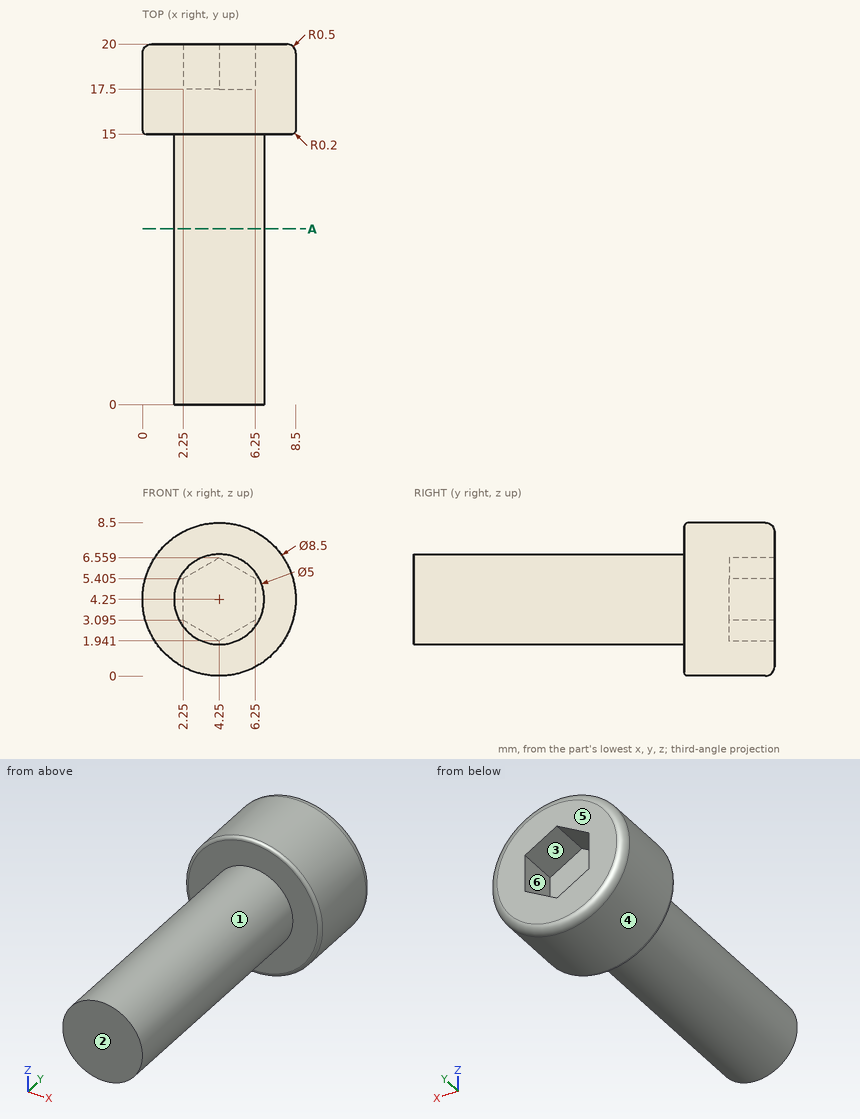
Could you check a few things on this drawing? It's one solid part, dimensions in mm from its lowest x, y, z. A direction names the side the tool comes from. Give positions to 0.01 mm unless a question says otherwise; leave off trailing zeros. Write each loop counter-clockwise with the first axis right and the second up, starting at its lowest first coordinate (ties: lowest second). Pieces come first, ordered by that corner, then holes. Notation, with made-up numbers: (31.25, 84) - (71.25, 84) arc R26 cw to (71.25, 113) - close; hole circle Ø5 at (20.25, -8.5). An arc over 180 degrees is marked (long way). Use CSV: the item, a comma, the result in double quotes. Start each with the question number.
Item 1: For the marked faces 1, 2 and 3, which set-ups out of +Z, -Z, +X, -X, +Y, -Y let a thin tool reach every point of the face, with its end or its side?
Item 2: I want a section at A-A, the plane y = 9.75. Please give me the cut outline in (x, z).
Item 3: If I drill on line 1 along Y through (x, z) = (3.5, 2.5); line 2 along Z through (x, y) = (2.75, 6); line 3 along Y through (x, z) = (6, 6.75), over which ranges is the centre line in solid material (lowest first)?
Item 4: If we mould it in two halves opening along Z, with no side actions, what happens to the marked faces 4, 5 and 6? For each: pulls with the +Z half, pulls with the -Z half, needs draft (parallel to the pull), parting line crosses it, or undercut.
Item 5: I'm going to push flat-ended pins straight in: pin 1 (4 mm diameter, centred on y = 8, z = 7.5, fed in from -X) (1 decimal); pin 2 (5 mm diameter, centred on y = 3, z = 3.5, fed in from -X); pin 3 (3 mm diameter, centred on x = 7, y = 3.5, fed in from -Z) (1 decimal). Where does each tip first touch, or does it pass through?
Findings:
1,face 1,"-Y"
1,face 2,"+Z, -Z, +X, -X, -Y"
1,face 3,"+Y"
2,outline,"circle Ø5 at (4.25, 4.25)"
3,line 1,"y = 0 to 17.5"
3,line 2,"z = 2.25 to 6.25"
3,line 3,"y = 15 to 20"
4,face 4,"parting line crosses it"
4,face 5,"needs draft"
4,face 6,"undercut"
5,pin 1,"stops at x = 2.1"
5,pin 2,"stops at x = 1.75"
5,pin 3,"stops at z = 2.1"
